from build123d import *

# Parameters (mm, degrees)
BOSS_EXTRUDE1_DEPTH               = 101.6
SKETCH2_R                         = 38.1
CUT_EXTRUDE2_DEPTH                = 23.8125
F_1_4_20_TAPPED_HOLE1_D           = 5.1054
F_1_4_20_TAPPED_HOLE1_DEPTH       = 19.05
F_1_4_20_TAPPED_HOLE1_CBORE_D     = 6.35
F_1_4_20_TAPPED_HOLE1_CBORE_DEPTH = 12.7
F_1_4_20_TAPPED_HOLE1_TIP         = 1.533816902
H_0_266_DIAMETER_HOLE1_D          = 6.7564
F_1_4_20_TAPPED_HOLE2_AT_2_COUNT  = 2
F_1_4_20_TAPPED_HOLE2_AT_2_PITCH  = 12.7
CHAMFER1_SIZE                     = 2.54


with BuildPart() as part:
    # Sketch1 → Boss-Extrude1 (new body)
    with BuildSketch(Plane(origin=(0, 0, 0), x_dir=(1, 0, 0), z_dir=(0, 1, 0))):
        with BuildLine():
            Line((33.02, 64.77), (33.02, 48.193111541))
            ThreePointArc((33.02, 48.193111541), (58.42, 0), (33.02, -48.193111541))
            Line((33.02, -48.193111541), (33.02, -64.77))
            Line((33.02, -64.77), (83.82, -64.77))
            Line((83.82, -64.77), (83.82, 64.77))
            Line((83.82, 64.77), (33.02, 64.77))
        make_face()
    extrude(amount=BOSS_EXTRUDE1_DEPTH)

    # Sketch2 → Cut-Extrude2 (cut)
    with BuildSketch(Plane(origin=(83.82, 0, 0), x_dir=(0, 0, -1), z_dir=(1, 0, 0))):
        with Locations((0, 50.8)):
            Circle(SKETCH2_R)
    extrude(amount=-CUT_EXTRUDE2_DEPTH, mode=Mode.SUBTRACT)

    # 1/4-20 Tapped Hole1
    with Locations(Plane(origin=(83.82, 0, 0), x_dir=(0, 0, -1), z_dir=(1, 0, 0))):
        with Locations((-31.75, 82.55), (31.75, 82.55), (31.75, 19.05), (-31.75, 19.05)):
            CounterBoreHole(F_1_4_20_TAPPED_HOLE1_D / 2, F_1_4_20_TAPPED_HOLE1_CBORE_D / 2, F_1_4_20_TAPPED_HOLE1_CBORE_DEPTH, depth=F_1_4_20_TAPPED_HOLE1_DEPTH)
            with Locations((0, 0, -(F_1_4_20_TAPPED_HOLE1_DEPTH + F_1_4_20_TAPPED_HOLE1_TIP / 2))):  # 118° drill point
                Cone(0, F_1_4_20_TAPPED_HOLE1_D / 2, F_1_4_20_TAPPED_HOLE1_TIP, mode=Mode.SUBTRACT)

    # H (0.266) Diameter Hole1 (through all)
    with Locations(Plane(origin=(0, 101.6, 0), x_dir=(-1, 0, 0), z_dir=(0, 1, 0))):
        with Locations((76.2, -57.15), (76.2, 57.15), (-76.2, 57.15), (-76.2, -57.15)):
            Hole(H_0_266_DIAMETER_HOLE1_D / 2)

    # Sketch11 → 1/4-20 Tapped Hole2 (revolve, cut)
    with BuildSketch(Plane(origin=(64.77, 82.20380383, 64.77), x_dir=(0, -1, 0), z_dir=(1, 0, 0))):
        Polygon((0, 0), (0, 20.583816902), (2.5527, 19.05), (2.5527, 12.7), (3.175, 12.7), (3.175, 0), align=None)
    f_1_4_20_tapped_hole2 = revolve(axis=Axis((64.77, 82.20380383, 71.12), (0, 0, -1)), mode=Mode.SUBTRACT)

    # 1/4-20 Tapped Hole2 at 2: 1/4-20 Tapped Hole2 ×2
    with Locations(*[(-i * F_1_4_20_TAPPED_HOLE2_AT_2_PITCH, 0, 0) for i in range(1, F_1_4_20_TAPPED_HOLE2_AT_2_COUNT)]):
        add(f_1_4_20_tapped_hole2, mode=Mode.SUBTRACT)

    # Mirror1: 1/4-20 Tapped Hole2 across plane
    add(f_1_4_20_tapped_hole2.mirror(Plane.XY), mode=Mode.SUBTRACT)

    # Mirror1 copy 1 sketch → Mirror1 copy 1 (revolve, cut)
    with BuildSketch(Plane(origin=(52.07, 82.20380383, -64.77), x_dir=(0, -1, 0), z_dir=(1, 0, 0))):
        Polygon((0, 0), (0, -20.583816902), (2.5527, -19.05), (2.5527, -12.7), (3.175, -12.7), (3.175, 0), align=None)
    revolve(axis=Axis((52.07, 82.20380383, -71.12), (0, 0, -1)), mode=Mode.SUBTRACT)

    # Chamfer1
    chamfer1_edges = [part.edges().sort_by_distance(p)[0] for p in [
        (83.82, 50.8, 64.77),
        (83.82, 50.8, -64.77),
        (58.42, 101.6, 64.77),
        (83.82, 101.6, 0),
        (58.42, 101.6, -64.77),
    ]]
    chamfer(chamfer1_edges, length=CHAMFER1_SIZE)


solid = part.part
Can you work these out from the model? Positions are in its coordinate system, mm. A direction names the side the tool comes from. Give positions to 0.01 mm unless a question says otherwise; leave off trailing zeros. Order: outer loops, then holes, each group sorted by start corner. A loop starts at its lowest first (then second) coordinate and runs counter-clockwise, first axis right, second up. Notation, with made-up numbers: M 67.25,-5.5 L 83.25,-5.5 A18 ccw 83.25,0.5 Z; hole C 67,85 d10. An arc over 180 degrees is marked long. Use one line per item in the form item = value. Start each with the question number.
Item 1: Will these pins go through, and if not, where does the flat tip stop? pin 1 Ø4 at (y, z) = (19.05, 31.75) entering from +X; pin 2 Ø4 at (y, z) = (82.55, -31.75) entering from -X; pin 3 Ø5.5 at (y, z) = (82.55, 31.75) entering from +X.
Item 2: For faces 1 (the cylindrical face through (54.56, 82.76, 48.94)), 2 (the flat face through (33.02, 50, -57)), 3 (the cylindrical face through (67.901, 80.285, 32.928)), 4 (the cylindrical face through (51.116, 79.175, -58.509)), which set-ups out of +Z, -Z, +X, -X, +Y, -Y let a thin tool reach every point of the face, with its end or its side?
Item 3: If I drill on line 1 along Y through (x, z) = (78, 0); line 2 along Z through (x, y) = (68, 19) (3 decimals); line 3 along Y through (x, z) = (52.07, -48.75), over which ranges is the centre line in solid material (lowest first)?
Item 4: We'd pull the mould along X, two halves only. Please class faces 5 (the conical face through (65.04, 82.556, 44.453)), 6 (the cylindrical face through (77.56, 15.95, 32.44)), 7 (the cylindrical face through (58.415, 50.089, -0.793)): +X half, -X half, draft (parallel to the pull), parting line (faces both ways), or undercut.
Item 5: If we section it at B-B (y = 92.5): Write out the boundary of the cut face in (x, z), then the cut area to 3 significant figures.
Item 6: If we section it at D-D (z = -14): Write out the boundary of the cut face in (x, y).
Item 7: If we section it at A-A (x = 76.2): Write out the boundary of the cut face in (y, z) (3 decimals).
Item 8: If we section it at C-C (x = 39.5): Write out the boundary of the cut face in (y, z).
Outcome:
q1.pin_1 = 64.44
q1.pin_2 = 47.68
q1.pin_3 = 71.12
q2.face_1 = +Z
q2.face_2 = +Z, -Z, -X, +Y, -Y
q2.face_3 = +X
q2.face_4 = -Z
q3.line_1 = 0 to 12.7, 88.9 to 101.6
q3.line_2 = -64.77 to -34.302, -29.198 to -20.985, 20.985 to 29.198, 34.302 to 64.77
q3.line_3 = 0 to 79.65, 84.76 to 101.6
q4.face_5 = undercut
q4.face_6 = draft
q4.face_7 = -X half
q5.outline = M 33.02,-64.77 L 81.28,-64.77 L 83.82,-62.23 L 83.82,62.23 L 81.28,64.77 L 33.02,64.77 L 33.02,48.19 A58.42 cw 33.02,-48.19 Z; hole C 76.2,-57.15 d6.76; hole C 76.2,57.15 d6.76
q5.area = 4,780 mm2
q6.outline = M 56.72,0 L 83.82,0 L 83.82,15.37 L 60.01,15.37 L 60.01,86.23 L 83.82,86.23 L 83.82,99.06 L 81.28,101.6 L 56.72,101.6 Z
q7.outline = M 0,-64.77 L 99.06,-64.77 L 101.6,-62.23 L 101.6,-60.528 L 0,-60.528 Z; M 0,-53.772 L 101.6,-53.772 L 101.6,53.772 L 0,53.772 Z; M 0,60.528 L 101.6,60.528 L 101.6,62.23 L 99.06,64.77 L 0,64.77 Z; hole C 50.8,0 d76.2; hole C 19.05,-31.75 d6.35; hole C 19.05,31.75 d6.35; hole C 82.55,-31.75 d6.35; hole C 82.55,31.75 d6.35
q8.outline = M 0,-64.77 L 99.06,-64.77 L 101.6,-62.23 L 101.6,-43.04 L 0,-43.04 Z; M 0,43.04 L 101.6,43.04 L 101.6,62.23 L 99.06,64.77 L 0,64.77 Z
